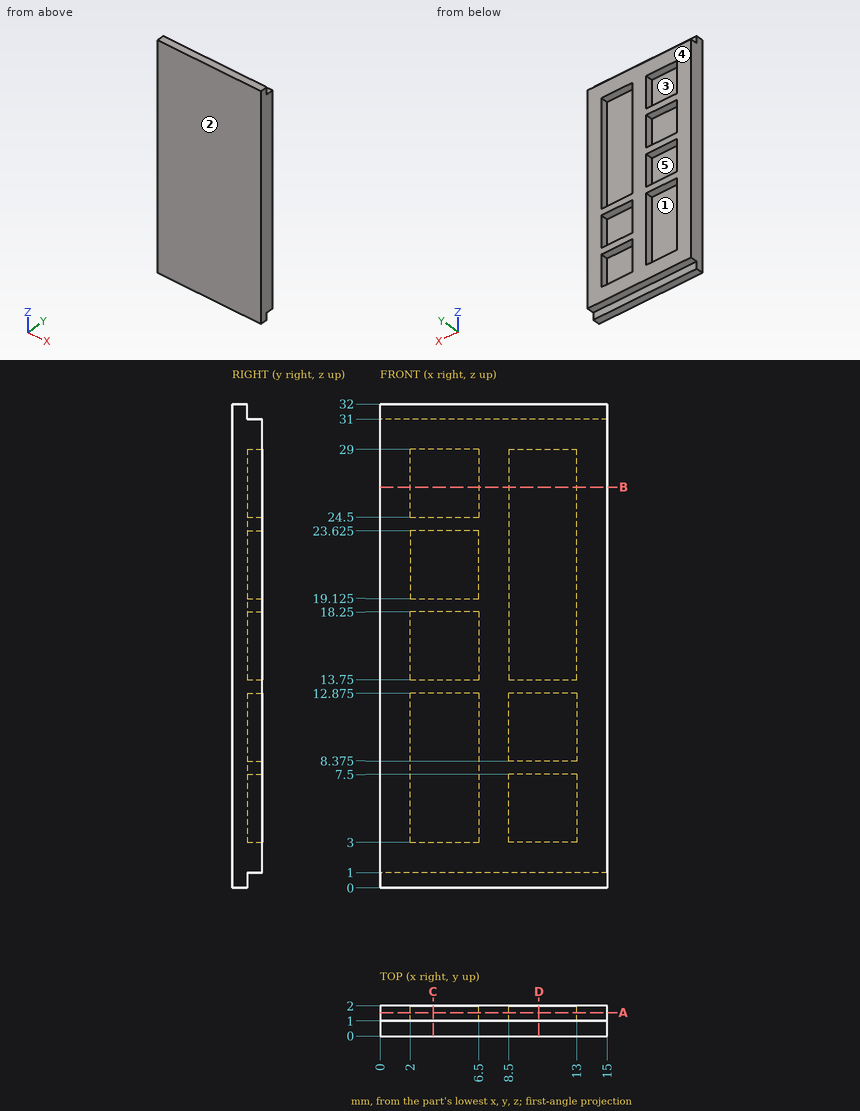
Geometry check sheet. Reference: drawing and pictorial views, mm from the part's lowest x, y, z. A direction names the side the tool comes from. Round coordinates to 2 decimals unless told otherwise and drop trailing zeros. Write each loop counter-clockwise with the first axis right and the second up, starting at its lowest first coordinate (ties: lowest second). Pieces come first, ordered by that corner, then holes. Notation, with made-up numbers: (77, 52) -> (129, 52) arc R14 cw to (129, 67) -> close; hole circle Ø1 at (86.25, -19). An arc over 180 degrees is marked (long way). Put each result on its own line as item: value.
1) Cross-section at D-D, the plane x = 10.5. Enter the section's corners in (y, z) (3 decimals), plus the area to 4 significant figures.
Recorded:
outline: (0, 0) -> (1, 0) -> (1, 1) -> (2, 1) -> (2, 3) -> (1, 3) -> (1, 7.5) -> (2, 7.5) -> (2, 8.375) -> (1, 8.375) -> (1, 12.875) -> (2, 12.875) -> (2, 13.75) -> (1, 13.75) -> (1, 29) -> (2, 29) -> (2, 31) -> (1, 31) -> (1, 32) -> (0, 32) -> close
area: 37.75 mm2
2) Access from +Z, -Z, +X, -X, +Y, -Y to the whole of each face (thin tool, end or side, straight path). Record for the marked faces 4 and 5.
Recorded:
face 4: +Z, -Z, +X, -X, +Y
face 5: +Y
3) Release check for a two-part mould opening along Z. For the marked faces 1, 2 and 3 record: pulls with the +Z half, pulls with the -Z half, needs draft (parallel to the pull), parting line crosses it, or undercut.
Recorded:
face 1: undercut
face 2: needs draft
face 3: undercut
4) Cross-section at B-B, the plane z = 26.5. Enter the section's corners in (x, y), plus the area to 3 significant figures.
Recorded:
outline: (0, 0) -> (15, 0) -> (15, 2) -> (13, 2) -> (13, 1) -> (8.5, 1) -> (8.5, 2) -> (6.5, 2) -> (6.5, 1) -> (2, 1) -> (2, 2) -> (0, 2) -> close
area: 21.0 mm2
5) Thickness scan on probe 1 along Z at (x, y) = (11.75, 1.4) (3 decimals); probe 2 along Z at (x, y) = (2.25, 1.65) (3 decimals); probe 3 along X at (y, z) = (1.6, 4). Record the ranges inside material, lowest first. Write a range as from..to.
Recorded:
probe 1: z = 1..3, 7.5..8.375, 12.875..13.75, 29..31
probe 2: z = 1..3, 12.875..13.75, 18.25..19.125, 23.625..24.5, 29..31
probe 3: x = 0..2, 6.5..8.5, 13..15
6) Cross-section at A-A, the plane y = 1.55. Give the number of separate pieces and of enclosed holes in the cut face, plus the area to 3 significant figures.
Recorded:
separate pieces: 1
enclosed holes: 7
area: 236 mm2
7) Cross-section at C-C, the plane x = 3.5. Enter the section's corners in (y, z) (3 decimals).
Recorded:
outline: (0, 0) -> (1, 0) -> (1, 1) -> (2, 1) -> (2, 3) -> (1, 3) -> (1, 12.875) -> (2, 12.875) -> (2, 13.75) -> (1, 13.75) -> (1, 18.25) -> (2, 18.25) -> (2, 19.125) -> (1, 19.125) -> (1, 23.625) -> (2, 23.625) -> (2, 24.5) -> (1, 24.5) -> (1, 29) -> (2, 29) -> (2, 31) -> (1, 31) -> (1, 32) -> (0, 32) -> close
8) Depth check by flat-ended pin: P1, Ø0.5, axis at x = 11, y = 1.5, coming from the +Z side; P2, Ø0.5, axis at x = 8, z = 31.5, coming from the +Y side; P3, Ø0.5, axis at x = 4, y = 1.5, coming from the -Z side. Enter the tip coordinate at first touch or a pass-through.
Recorded:
P1: stops at z = 31
P2: stops at y = 1
P3: stops at z = 1
